Autodesk Inventor part; units mm, degrees
ref_plane "YZ Plane" through (0, 0, 0) normal (1, 0, 0) x (0, 1, 0)
ref_plane "XZ Plane" through (0, 0, 0) normal (0, 1, 0) x (-1, 0, 0)
ref_plane "XY Plane" through (0, 0, 0) normal (0, 0, 1) x (1, 0, 0)
sketch "Sketch1" plane through (0, 0, 0) normal (0, 0, 1) x (1, 0, 0)
  line L0 (-750, 67.6691) -> (750, 67.6691)
  line L1 (750, 67.6691) -> (750, 0)
  line L2 (750, 0) -> (-750, 0)
  line L3 (-750, 0) -> (-750, 67.6691)
  point P0 (0, 0)
  point P1 (0, 0)
  dimension "d0" = 1500
  dimension "d1" = 67.669
extrude "Plate1" add sketch "Sketch1" along normal blind 2
sketch "Sketch2" plane through (750, 2, 0) normal (0, -1, 0) x (1, 0, 0)
  line L0 (-1500, 0) -> (0, 0)
  line L1 (0, 0) -> (0, 30)
  line L2 (0, 30) -> (-1500, 30)
  line L3 (-1500, 30) -> (-1500, 0)
edge flange "Flange1" height 30 angle 90 thickness 2 bend radius 2.75 thickness toward (0, -1, 0) relief round relief width 2 relief depth 1 edges at (0, 0, 2) wall of the first edge with corners at (-750, 2, 0) (750, 2, 0) (750, 2, 30) (-750, 2, 30)
bend "Bend1"
corner "Corner1"
sketch "Sketch6" plane through (0, 0, 0) normal (0, 0, -1) x (-1, 0, 0)
  line L0 (-750, 67.6691) -> (-750, 4.75)
  circle A0 centre (-750, 67.6691) radius 22.5
  line L1 (-750, 67.6691) -> (750, 67.6691)
  line L2 (-1, 67.6691) -> (-1, 30)
  line L3 (-499, 30) -> (-499, 67.6691)
  line L4 (-1, 30) -> (-499, 30) construction
  circle A1 centre (-250, 67.6691) radius 22.5
  point P0 (0, 0)
  point P1 (-727.5, 67.6691)
  point P2 (-750, 45.1691)
  point P3 (-250, 30)
  dimension "d24" = 45
extrude "Extrusion2" cut sketch "Sketch6" along normal mid plane 30 contours L1 A0 L0 picked at (-748.3311, 52.8571)
sketch "Sketch7" plane through (0, 0, 2) normal (0, 0, 1) x (1, 0, 0)
  line L0 (-750, 4.75) -> (-750, 67.6691)
  line L1 (-750, 4.75) -> (750, 4.75)
  line L2 (750, 45.1691) -> (750, 4.75)
  arc A0 (727.5, 67.6691) -> (750, 45.1691) centre (750, 67.6691) ccw
  line L3 (-750, 67.6691) -> (727.5, 67.6691)
  line L4 (649, 32.2095) -> (651, 32.2095)
  line L5 (651, 32.2095) -> (651, 40.2095)
  line L6 (651, 40.2095) -> (649, 40.2095)
  line L7 (649, 40.2095) -> (649, 32.2095)
  line L8 (-750, 4.75) -> (750, 4.75)
  line L9 (650, 4.75) -> (650, 67.6691) construction
  line L10 (637, 32.2095) -> (639, 32.2095)
  line L11 (639, 32.2095) -> (639, 40.2095)
  line L12 (639, 40.2095) -> (637, 40.2095)
  line L13 (637, 40.2095) -> (637, 32.2095)
  point P0 (0, 0)
  point P1 (650, 32.2095)
  point P2 (649, 36.2095)
  point P3 (650, 36.2095)
  point P4 (639, 36.2095)
  dimension "d30" = 2
  dimension "d31" = 8
  dimension "d32" = 100
  dimension "d33" = 2
  dimension "d34" = 8
  dimension "d35" = 10
extrude "Extrusion3" [suppressed]
mirror "Mirror2" [suppressed]
sketch "Sketch9" plane through (0, 0, 2) normal (0, 0, 1) x (1, 0, 0)
  line L0 (494, 62.6691) -> (494, 50.6691) construction
  line L1 (494, 50.6691) -> (294, 50.6691) construction
  line L2 (294, 50.6691) -> (294, 62.6691) construction
  line L3 (294, 62.6691) -> (494, 62.6691) construction
  line L4 (499, 30) -> (499, 67.6691)
  line L5 (-750, 67.6691) -> (750, 67.6691)
  point P0 (0, 0)
  point P1 (1, 67.6691)
  dimension "d40" = 200
  dimension "d41" = 12
  dimension "d42" = 5
  dimension "d43" = 5
mark "Mark2"
equation "\"d1\" = Стрингер_2"
equation "\"d43\" = d42"
equation "\"d2\" = Thickness"
equation "\"d3\" = BendReliefWidth"
equation "\"d4\" = BendReliefDepth"
equation "\"d5\" = MinimumRemnant"
equation "\"d6\" = TransitionRadius"
equation "\"d9\" = BendRadius"
equation "\"d10\" = CornerReliefSize"
equation "\"d11\" = GapSize"
equation "\"d12\" = JacobiRadiusSize"
equation "\"BendReliefWidth\" = Thickness"
equation "\"BendReliefDepth\" = 0.5 * Thickness"
equation "\"CornerReliefSize\" = 4 * Thickness"
equation "\"MinimumRemnant\" = 2 * Thickness"
equation "\"TransitionRadius\" = BendRadius"
equation "\"JacobiRadiusSize\" = BendRadius"
equation "\"GapSize\" = Thickness"
equation "\"qqqqqq\" = 67.35706"
properties part number "МОО 068 stringer lowerback" material "Stainless Steel"
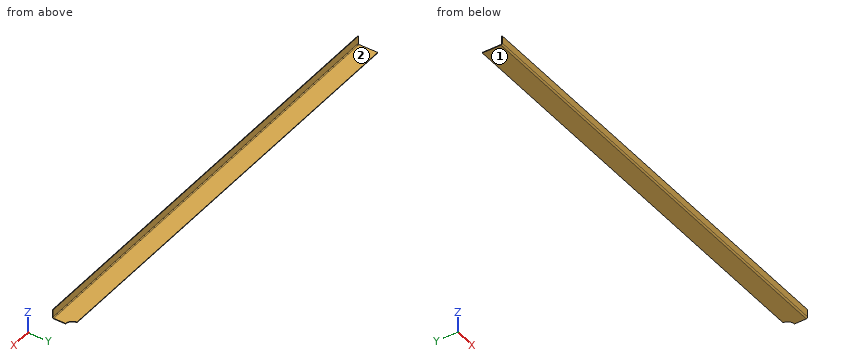
Verification items for the finished model (mm, model axes). Face numbers are marked on the shaded views. A direction names the side the tool comes from. Give positions to 0.01 mm unless a question says otherwise; leave off trailing zeros. Order: outer loops, then holes, each group sorted by start corner. A loop starts at its lowest first (then second) coordinate and runs counter-clockwise, first axis right, second up. Notation, with made-up numbers: (5.5, 67.5) -> (47.5, 67.5) arc R31 ccw to (47.5, 105.5) -> close; hole circle Ø8 at (74, 83.25). An arc over 180 degrees is marked (long way). Answer as CSV lines item,"result".
Q1. Sectioned sample at A-A on x = 245. Record the cut outline in (y, z), plus the area to 3 significant figures.
Solutions:
outline,"(0, 4.75) arc R4.75 ccw to (4.75, 0) -> (67.67, 0) -> (67.67, 2) -> (4.75, 2) arc R2.75 cw to (2, 4.75) -> (2, 30) -> (0, 30) -> close"
area,"188 mm²"
Q2. Sectioned sample at B-B on y = 32. Record the cut outline in (x, z).
Solutions:
outline,"(-750, 0) -> (750, 0) -> (750, 2) -> (-750, 2) -> close"
Q3. Depth check by flat-ended pin: pin 1 (2 mm diameter, centred on x = -378.5, z = 19.5, fed in from -Y); pin 2 (1.5 mm diameter, centred on x = 179, z = 8.5, fed in from +Y); pin 3 (6 mm diameter, centred on x = -103, z = 7, fed in from +Y); pin 4 (19 mm diameter, centred on x = -212, y = 28, fed in from +Z). Enter the tip coordinate at first touch or a pass-through.
Solutions:
pin 1,"stops at y = 0"
pin 2,"stops at y = 2"
pin 3,"stops at y = 2.1"
pin 4,"stops at z = 2"
Q4. Access from +Z, -Z, +X, -X, +Y, -Y to the whole of each face (thin tool, end or side, straight path). Record for the marked faces 1 and 2.
Solutions:
face 1,"-Z, +X, -X, +Y, -Y"
face 2,"+Z, +X, -X, +Y"
Q5. Scan lines: probe 1 along Z at (x, y) = (394, 44.5); probe 2 along Y at (x, z) = (-69, 4). Record each from-to range of solid material in increasing order.
Solutions:
probe 1,"z = 0 to 2"
probe 2,"y = 0.06 to 2.1"
